```python
from build123d import *

# Parameters (mm, degrees)
SKETCH1_W           = 82
SKETCH1_H           = 153
BOSS_EXTRUDE1_DEPTH = 420
SHELL1_T            = -1.5
SKETCH4_R           = 3
CUT_EXTRUDE1_DEPTH  = 154
CUT_EXTRUDE2_REACH  = 436.714
SKETCH5_R           = 3


with BuildPart() as part:
    # Sketch1 → Boss-Extrude1 (new body)
    with BuildSketch(Plane.XY):
        Rectangle(SKETCH1_W, SKETCH1_H)
    extrude(amount=BOSS_EXTRUDE1_DEPTH)

    # Shell1
    shell1_openings = [part.faces().sort_by_distance(p)[0] for p in [
        (0, 0, 420),
        (0, 0, 0),
        (41, 0, 210),
    ]]
    offset(amount=SHELL1_T, openings=shell1_openings, kind=Kind.INTERSECTION)

    # Sketch4 → Cut-Extrude1 (cut)
    with BuildSketch(Plane(origin=(0, 76.5, 0), x_dir=(1, 0, 0), z_dir=(0, 1, 0))):
        with Locations(Location((-0.5, -8, 0), (0, 0, 180))):
            Circle(SKETCH4_R)
        with Locations((-0.5, -412)):
            Circle(SKETCH4_R)
    extrude(amount=-CUT_EXTRUDE1_DEPTH, mode=Mode.SUBTRACT)

    # Sketch5 → Cut-Extrude2 (cut, up to next)
    with BuildSketch(Plane.ZY.offset(41), mode=Mode.PRIVATE) as cut_extrude2_sk1:
        with Locations((8, 0)):
            Circle(SKETCH5_R)
    cut_extrude2_tool1 = extrude(cut_extrude2_sk1.sketch, amount=-CUT_EXTRUDE2_REACH, mode=Mode.PRIVATE) & part.part
    # Sketch5 → Cut-Extrude2 (cut, up to next)
    with BuildSketch(Plane.ZY.offset(41), mode=Mode.PRIVATE) as cut_extrude2_sk2:
        with Locations((412, 0)):
            Circle(SKETCH5_R)
    cut_extrude2_tool2 = extrude(cut_extrude2_sk2.sketch, amount=-CUT_EXTRUDE2_REACH, mode=Mode.PRIVATE) & part.part
    add(cut_extrude2_tool1.solids().sort_by_distance((-41, 0, 8))[0], mode=Mode.SUBTRACT)
    add(cut_extrude2_tool2.solids().sort_by_distance((-41, 0, 412))[0], mode=Mode.SUBTRACT)


solid = part.part
```
Read the model definition and answer for the solid it produces. Units are mm, in the model's axes. A direction names the side the tool comes from. Round coordinates to 2 decimals unless told otherwise and drop trailing zeros. Write each loop counter-clockwise with the first axis right and the second up, starting at its lowest first coordinate (ties: lowest second). Pieces come first, ordered by that corner, then holes. Notation, with made-up numbers: (37, 10) - (42, 10) arc R14 ccw to (42, 24) - close; hole circle Ø7 at (50, 9). An arc over 180 degrees is marked (long way). Use CSV: the item, a comma, the result in double quotes.
Q1. Find section A-A, the plane x = 33. Write down the section's boundary in (y, z).
Values:
outline,"(-76.5, 0) - (-75, 0) - (-75, 420) - (-76.5, 420) - close; (75, 0) - (76.5, 0) - (76.5, 420) - (75, 420) - close"
Q2. Find section C-C, the plane y = -9. Write down the section's boundary in (x, z).
Values:
outline,"(-41, 0) - (-39.5, 0) - (-39.5, 420) - (-41, 420) - close"
Q3. Straight lines are drawn through the part: line 1 along Z through (x, y) = (-0.5, -75.85); line 2 along Y through (x, z) = (-40.05, 412); line 3 along Y through (x, z) = (-15.5, 139). For each, find the intervals that lie inside material, in ascending order.
Values:
line 1,"z = 0 to 5, 11 to 409, 415 to 420"
line 2,"y = -76.5 to -3, 3 to 76.5"
line 3,"y = -76.5 to -75, 75 to 76.5"
Q4. A tool of negligible diameter and unlimited length cuts with its end or side. For faces 1 (the flat face through (-1, 76.5, 207)), 2 (the flat face through (0, 75, 207)), from which of +Z, -Z, +X, -X, +Y, -Y can it reach the whole face along a straight path? Write none if from no direction.
Values:
face 1,"+Z, -Z, +X, -X, +Y"
face 2,"+Z, -Z, +X"
Q5. Each of these flat-tipped pins is pushed along its axis until it touches: pin 1 Ø5 at (y, z) = (56, 283.5) entering from +X; pin 2 Ø9.5 at (y, z) = (0, 412) entering from -X. Where does it stop, or does it pass through?
Values:
pin 1,"stops at x = -39.5"
pin 2,"stops at x = -41"
Q6. Determine the mould class of faces 3 (the flat face through (-41, -1, 207)), 4 (the flat face through (-39.5, -1, 207)), 5 (the flat face through (-1, -76.5, 207)), 6 (the flat face through (0, -75, 207)) for opening direction Y: +Y half, -Y half, draft (parallel to the pull), parting line (faces both ways), or undercut.
Values:
face 3,"draft"
face 4,"undercut"
face 5,"-Y half"
face 6,"undercut"
Q7. Find section B-B, the plane z = 368. Write down the section's boundary in (x, y).
Values:
outline,"(-41, -76.5) - (41, -76.5) - (41, -75) - (-39.5, -75) - (-39.5, 75) - (41, 75) - (41, 76.5) - (-41, 76.5) - close"
